```python
from build123d import *

# Parameters (mm, degrees)
SKETCH4_W              = 76.2
SKETCH4_H              = 44.45
BASE_FLANGE1_DEPTH     = 1.905
SKETCHED_START         = -38.1
SKETCHED_BEND3_DEPTH   = 76.2
SKETCHED_BEND3_2_DEPTH = 76.2
CUT_EXTRUDE2_REACH     = 49.608
SKETCH20_R             = 2


# Read off the part's stored shape, not the designer's step: Sketched Bend3
# Sheet-metal steps are written as plain solids
with BuildPart() as part:
    # Sketch4 → Base-Flange1 (new body)
    with BuildSketch(Plane(origin=(0, 0, 0), x_dir=(0, 0, -1), z_dir=(1, 0, 0))):
        Rectangle(SKETCH4_W, SKETCH4_H)
    extrude(amount=-BASE_FLANGE1_DEPTH)

    # Sketched Bend3 outline → Sketched Bend3 (cut)
    with BuildSketch(Plane.XY.offset(SKETCHED_START)):
        with BuildLine():
            ThreePointArc((0, -13.357223013), (-1.375727285, -12.406629491), (-1.905, -10.8204))
            Line((-1.905, -10.8204), (-1.905, -22.225))
            Line((-1.905, -22.225), (0, -22.225))
            Line((0, -22.225), (0, -13.357223013))
        make_face()
        with BuildLine():
            Line((-1.905, 22.225), (-1.905, 10.8204))
            ThreePointArc((-1.905, 10.8204), (-1.375727285, 12.406629491), (0, 13.357223013))
            Line((0, 13.357223013), (0, 22.225))
            Line((0, 22.225), (-1.905, 22.225))
        make_face()
    extrude(amount=SKETCHED_BEND3_DEPTH, mode=Mode.SUBTRACT)

    # Sketched Bend3 2 outline → Sketched Bend3 2 (add)
    with BuildSketch(Plane.XY.offset(SKETCHED_START)):
        with BuildLine():
            Line((0, -10.8204), (0, -13.357223013))
            ThreePointArc((0, -13.357223013), (0.364592683, -13.435674577), (0.7366, -13.462))
            Line((0.7366, -13.462), (9.487967924, -13.462))
            Line((9.487967924, -13.462), (9.487967924, -11.557))
            Line((9.487967924, -11.557), (0.7366, -11.557))
            ThreePointArc((0.7366, -11.557), (0.215745145, -11.341254855), (0, -10.8204))
        make_face()
        with BuildLine():
            ThreePointArc((0.7366, 13.462), (0.364592683, 13.435674577), (0, 13.357223013))
            Line((0, 13.357223013), (0, 10.8204))
            ThreePointArc((0, 10.8204), (0.215745145, 11.341254855), (0.7366, 11.557))
            Line((0.7366, 11.557), (9.487967924, 11.557))
            Line((9.487967924, 11.557), (9.487967924, 13.462))
            Line((9.487967924, 13.462), (0.7366, 13.462))
        make_face()
    extrude(amount=SKETCHED_BEND3_2_DEPTH)

    # Cut-Extrude2: up to this face of the body (flat: up to its plane)
    cut_extrude2_end = Plane(part.part.faces().sort_by_distance((5.112283962, -13.462, 0))[0])
    # Sketch20 → Cut-Extrude2 (cut, up to the picked face)
    with BuildSketch(Plane(origin=(0, 13.462, 0), x_dir=(1, 0, 0), z_dir=(0, 1, 0)), mode=Mode.PRIVATE) as cut_extrude2_sk1:
        with Locations(Location((5.08, -3.175, 0), (0, 0, 180))):
            Circle(SKETCH20_R)
    cut_extrude2_tool1 = split(extrude(cut_extrude2_sk1.sketch, amount=-CUT_EXTRUDE2_REACH, mode=Mode.PRIVATE), bisect_by=cut_extrude2_end, keep=Keep.BOTH, mode=Mode.PRIVATE)
    # Sketch20 → Cut-Extrude2 (cut, up to the picked face)
    with BuildSketch(Plane(origin=(0, 13.462, 0), x_dir=(1, 0, 0), z_dir=(0, 1, 0)), mode=Mode.PRIVATE) as cut_extrude2_sk2:
        with Locations(Location((5.08, 3.175, 0), (0, 0, 180))):
            Circle(SKETCH20_R)
    cut_extrude2_tool2 = split(extrude(cut_extrude2_sk2.sketch, amount=-CUT_EXTRUDE2_REACH, mode=Mode.PRIVATE), bisect_by=cut_extrude2_end, keep=Keep.BOTH, mode=Mode.PRIVATE)
    # Sketch20 → Cut-Extrude2 (cut, up to the picked face)
    with BuildSketch(Plane(origin=(0, 13.462, 0), x_dir=(1, 0, 0), z_dir=(0, 1, 0)), mode=Mode.PRIVATE) as cut_extrude2_sk3:
        with Locations(Location((5.08, 9.525, 0), (0, 0, 180))):
            Circle(SKETCH20_R)
    cut_extrude2_tool3 = split(extrude(cut_extrude2_sk3.sketch, amount=-CUT_EXTRUDE2_REACH, mode=Mode.PRIVATE), bisect_by=cut_extrude2_end, keep=Keep.BOTH, mode=Mode.PRIVATE)
    # Sketch20 → Cut-Extrude2 (cut, up to the picked face)
    with BuildSketch(Plane(origin=(0, 13.462, 0), x_dir=(1, 0, 0), z_dir=(0, 1, 0)), mode=Mode.PRIVATE) as cut_extrude2_sk4:
        with Locations(Location((5.08, 15.875, 0), (0, 0, 180))):
            Circle(SKETCH20_R)
    cut_extrude2_tool4 = split(extrude(cut_extrude2_sk4.sketch, amount=-CUT_EXTRUDE2_REACH, mode=Mode.PRIVATE), bisect_by=cut_extrude2_end, keep=Keep.BOTH, mode=Mode.PRIVATE)
    # Sketch20 → Cut-Extrude2 (cut, up to the picked face)
    with BuildSketch(Plane(origin=(0, 13.462, 0), x_dir=(1, 0, 0), z_dir=(0, 1, 0)), mode=Mode.PRIVATE) as cut_extrude2_sk5:
        with Locations(Location((5.08, -9.525, 0), (0, 0, 180))):
            Circle(SKETCH20_R)
    cut_extrude2_tool5 = split(extrude(cut_extrude2_sk5.sketch, amount=-CUT_EXTRUDE2_REACH, mode=Mode.PRIVATE), bisect_by=cut_extrude2_end, keep=Keep.BOTH, mode=Mode.PRIVATE)
    # Sketch20 → Cut-Extrude2 (cut, up to the picked face)
    with BuildSketch(Plane(origin=(0, 13.462, 0), x_dir=(1, 0, 0), z_dir=(0, 1, 0)), mode=Mode.PRIVATE) as cut_extrude2_sk6:
        with Locations(Location((5.08, -15.875, 0), (0, 0, 180))):
            Circle(SKETCH20_R)
    cut_extrude2_tool6 = split(extrude(cut_extrude2_sk6.sketch, amount=-CUT_EXTRUDE2_REACH, mode=Mode.PRIVATE), bisect_by=cut_extrude2_end, keep=Keep.BOTH, mode=Mode.PRIVATE)
    add(cut_extrude2_tool1.solids().sort_by(Axis((5.08, 13.462, 3.175), (0, -1, 0)))[0], mode=Mode.SUBTRACT)
    add(cut_extrude2_tool2.solids().sort_by(Axis((5.08, 13.462, -3.175), (0, -1, 0)))[0], mode=Mode.SUBTRACT)
    add(cut_extrude2_tool3.solids().sort_by(Axis((5.08, 13.462, -9.525), (0, -1, 0)))[0], mode=Mode.SUBTRACT)
    add(cut_extrude2_tool4.solids().sort_by(Axis((5.08, 13.462, -15.875), (0, -1, 0)))[0], mode=Mode.SUBTRACT)
    add(cut_extrude2_tool5.solids().sort_by(Axis((5.08, 13.462, 9.525), (0, -1, 0)))[0], mode=Mode.SUBTRACT)
    add(cut_extrude2_tool6.solids().sort_by(Axis((5.08, 13.462, 15.875), (0, -1, 0)))[0], mode=Mode.SUBTRACT)


solid = part.part
```
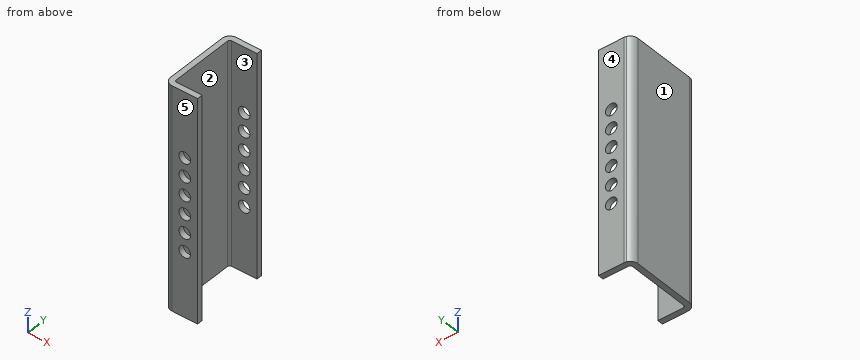
The model under review builds one solid part; all positions refer to its coordinate system, in mm. Face numbers are marked on the shaded views. A direction names the side the tool comes from. Round coordinates to 2 decimals unless told otherwise and drop trailing zeros. Loops run counter-clockwise (first coordinate to the right, second up) from the corner with the lowest first, then second, coordinate; pieces in that order, holes last.
1) Consider section D-D on x = 5.08. Give the number of separate pieces and of enclosed holes in the cut face, then the cut area to 3 significant figures.
Values follow:
separate pieces: 14
enclosed holes: 0
area: 199 mm2
2) Consider section C-C on y = 3.25. State the section outline as (x, z) points (3 decimals).
Values follow:
outline: (-1.905, -38.1) - (0, -38.1) - (0, 38.1) - (-1.905, 38.1) - close
3) Clearance check with a flat-ended pin moving along its axis: P1, Ø11, axis at y = -1.5, z = 12.5, coming from the +X side. State where the tip first meets the part, or that it passes through.
Values follow:
P1: stops at x = 0
4) The part is to be moulded in two halves that separate along Y. For the marked faces 3, 4 and 5, say which applies: pulls with the +Y half, pulls with the -Y half, needs draft (parallel to the pull), parting line crosses it, or undercut.
Values follow:
face 3: undercut
face 4: pulls with the +Y half
face 5: pulls with the -Y half
5) Consider section B-B on z = -32. State the section outline as (x, y) points (3 decimals).
Values follow:
outline: (-1.905, -10.82) arc R2.642 ccw to (0.737, -13.462) - (9.488, -13.462) - (9.488, -11.557) - (0.737, -11.557) arc R0.737 cw to (0, -10.82) - (0, 10.82) arc R0.737 cw to (0.737, 11.557) - (9.488, 11.557) - (9.488, 13.462) - (0.737, 13.462) arc R2.642 ccw to (-1.905, 10.82) - close
6) Consider section A-A on x = 1.5. State the section outline as (y, z) points.
Values follow:
outline: (-13.46, -38.1) - (-11.56, -38.1) - (-11.56, 38.1) - (-13.46, 38.1) - close; (11.56, -38.1) - (13.46, -38.1) - (13.46, 38.1) - (11.56, 38.1) - close
7) Tool access review of the marked faces 1 and 2: name each direction out of +Z, -Z, +X, -X, +Y, -Y from which nothing blocks a thin tool from reaching the whole face with its end or side.
Values follow:
face 1: +Z, -Z, -X, +Y, -Y
face 2: +Z, -Z, +X
8) Wall thickness on line 1 along Y through (x, z) = (6.75, -20); line 2 along X through (y, z) = (3, 35) (3 decimals); line 3 along X through (y, z) = (-12, -3): over which ranges is each line inside the solid? List them lowest first.
Values follow:
line 1: y = -13.46 to -11.56, 11.56 to 13.46
line 2: x = -1.905 to 0
line 3: x = -1.63 to 3.09, 7.07 to 9.49
